Autodesk Inventor part; units mm, degrees
ref_plane "YZ Plane" through (0, 0, 0) normal (1, 0, 0) x (0, 1, 0)
ref_plane "XZ Plane" through (0, 0, 0) normal (0, 1, 0) x (-1, 0, 0)
ref_plane "XY Plane" through (0, 0, 0) normal (0, 0, 1) x (1, 0, 0)
sketch "Sketch1" plane through (0, 0, 0) normal (0, 1, 0) x (-1, 0, 0)
  line L0 (0, 0) -> (609.6, 0)
  line L1 (609.6, 0) -> (609.6, -914.4)
  line L2 (609.6, -914.4) -> (0, -914.4)
  line L3 (0, -914.4) -> (0, 0)
  dimension "d0" = 609.6
  dimension "d1" = 914.4
extrude "Extrusion1" add sketch "Sketch1" along normal blind 152.4
shell "Shell1" thickness 12.7 removed faces 1 at (-203.2, 152.4, -304.8)
sketch "Sketch2" plane through (0, 0, -914.4) normal (0, 0, -1) x (-1, 0, 0)
  line L0 (596.9, 152.4) -> (12.7, 152.4)
  circle A0 centre (615.95, 152.4) radius 10.16
  circle A1 centre (615.95, 152.4) radius 6.35
  line L1 (609.6, 0) -> (609.6, 152.4)
  point P0 (0, 0)
  dimension "d5" = 12.7
  dimension "d6" = 20.32
  dimension "d7" = 6.35
extrude "Extrusion2" add sketch "Sketch2" against normal up to surface (914.4 mm away)
sketch "Sketch3" plane through (0, 152.4, 0) normal (0, 1, 0) x (1, 0, 0)
  point P0 (0, 0)
sketch "Sketch4" plane through (0, 0, 0) normal (1, 0, 0) x (0, 0, -1)
  line L0 (0, 0) -> (0, 152.4)
  line L1 (0, 152.4) -> (50.8, 152.4)
  line L2 (50.8, 152.4) -> (50.8, 178.2149)
  line L3 (50.8, 178.2149) -> (0, 178.2149)
  line L4 (0, 178.2149) -> (0, 152.4)
  line L5 (914.4, 152.4) -> (863.6, 152.4)
  line L6 (863.6, 152.4) -> (863.6, 178.2149)
  line L7 (863.6, 178.2149) -> (914.4, 178.2149)
  line L8 (914.4, 178.2149) -> (914.4, 152.4)
  line L9 (0, 152.4) -> (914.4, 152.4)
  line L10 (101.6, 152.4) -> (812.8, 152.4)
  line L11 (812.8, 152.4) -> (812.8, 202.1874)
  line L12 (812.8, 202.1874) -> (101.6, 202.1874)
  line L13 (101.6, 202.1874) -> (101.6, 152.4)
  dimension "d10" = 50.8
  dimension "d11" = 50.8
  dimension "d12" = 50.8
  dimension "d13" = 50.8
extrude "Extrusion3" cut sketch "Sketch4" against normal through all
sketch "Sketch5" plane through (0, 152.4, 0) normal (0, 1, 0) x (1, 0, 0)
  line L0 (-609.6, 0) -> (-609.6, 914.4)
  line L1 (-609.6, 0) -> (-640.6567, 0)
  line L2 (-640.6567, 0) -> (-640.6567, 50.8)
  line L3 (-640.6567, 50.8) -> (-609.6, 50.8)
  line L4 (-609.6, 50.8) -> (-609.6, 0)
  line L5 (-609.6, 101.6) -> (-609.6, 812.8)
  line L6 (-609.6, 101.6) -> (-640.6567, 101.6)
  line L7 (-640.6567, 101.6) -> (-640.6567, 812.8)
  line L8 (-640.6567, 812.8) -> (-609.6, 812.8)
  line L9 (-609.6, 812.8) -> (-609.6, 101.6)
  line L10 (-609.6, 863.6) -> (-609.6, 914.4)
  line L11 (-609.6, 863.6) -> (-644.9488, 863.6)
  line L12 (-644.9488, 863.6) -> (-644.9488, 914.4)
  line L13 (-644.9488, 914.4) -> (-609.6, 914.4)
  line L14 (-609.6, 914.4) -> (-609.6, 863.6)
  point P0 (0, 0)
extrude "Extrusion4" cut sketch "Sketch5" against normal blind 25.4
properties part number "chestLower"
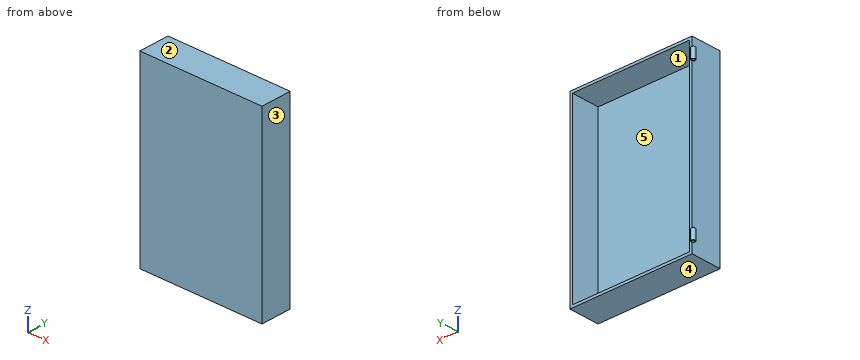
Geometry: final body of the model. Coordinates: model frame, mm. Face numbers are marked on the shaded views. A direction names the side the tool comes from. Coordinates: 2 decimals unless noted, no trailing zeros. Write each loop counter-clockwise with the first axis right and the second up, starting at its lowest first coordinate (ties: lowest second). Pieces come first, ordered by that corner, then holes. Notation, with made-up numbers: M -20.5,20.25 L 9.5,20.25 A25 ccw 9.5,48.25 Z; hole C 61.25,54 d11. An arc over 180 degrees is marked long. Answer as CSV lines item,"result". Start each with the question number.
Q1. Pin query (flat end, axial travel): P1, Ø12, axis at y = 52.5, z = -121, coming from the -X side; P2, Ø10, axis at x = -615.95, y = 152.4, coming from the +Z side. Return the tip coordinate at first contact, or that it passes through.
Q2. Mould query, pull axis Z, two halves, no side actions, for the marked faces 3, 4 and 5. Classes: released by +Z, released by -Z, zero draft, split by the parting line, or undercut.
Q3. Cut plane B-B on z = -381. Return the cut outline in (x, y).
Q4. Line query: line 1 (Y direction, x = -615.95, z = -824); line 2 (X direction, y = 79.5, z = -615); line 3 (X direction, y = 152, z = -833). Output: solid intervals per line, ascending. Write a range as from..to.
Q5. Reachability of the marked faces 1 and 2 from +Z, -Z, +X, -X, +Y, -Y: full face, straight path, thin tool, end or side. Return the list, or none.
Q6. Cut plane C-C on x = -244. Return the cut outline in (y, z).
Q7. Cut plane A-A on y = 54. Return the cut outline in (x, z).
Findings below:
1,P1,"stops at x = -609.6"
1,P2,"passes through"
2,face 3,"zero draft"
2,face 4,"released by -Z"
2,face 5,"undercut"
3,outline,"M -609.6,0 L 0,0 L 0,152.4 L -12.7,152.4 L -12.7,12.7 L -596.9,12.7 L -596.9,152.4 L -609.6,152.4 Z"
4,line 1,"y = 142.24..146.05, 158.75..162.56"
4,line 2,"x = -609.6..-596.9, -12.7..0"
4,line 3,"x = -626.1..-622.29, -609.61..-596.9, -12.7..0"
5,face 1,"+Y"
5,face 2,"+Z, +X, -X, +Y, -Y"
6,outline,"M 0,-914.4 L 152.4,-914.4 L 152.4,-901.7 L 12.7,-901.7 L 12.7,-12.7 L 152.4,-12.7 L 152.4,0 L 0,0 Z"
7,outline,"M -609.6,-914.4 L 0,-914.4 L 0,0 L -609.6,0 Z; hole M -596.9,-901.7 L -12.7,-901.7 L -12.7,-12.7 L -596.9,-12.7 Z"
